```python
from build123d import *

# Parameters (mm, degrees)
F0_W        = 50.8
F0_H        = 26.0105735242
F1_DEPTH    = 6.35
F2_W        = 50.6046172231
F2_H        = 51.1175021529
F3_DEPTH    = 25.4
F4_T4_DEPTH = 51.1175021529
F4_T9_DEPTH = 64.038633205
F5_SIZE     = 5.08


# Not quite as in the source:
# - a fillet or chamfer that OpenCascade refuses, or shapes differently, is made with other operations: its cross-section is extruded or revolved along the edge and cut away or added


with BuildPart() as f1:
    # F0 (on Front) → F1 (new body)
    with BuildSketch(Plane.XZ):
        with Locations((0, -37.7947132379)):
            Rectangle(F0_W, F0_H)
        Polygon((-38.1, -24.7894264758), (-25.4, -24.7894264758), (-25.4, 0), align=None)
        Polygon((25.4, -50.8), (-25.4, -50.8), (-25.4, -24.7894264758), (-38.1, -24.7894264758), (-38.1, -51.4594204724), (38.1, -51.4594204724), (38.1, -24.7894264758), (25.4, -24.7894264758), align=None)
        Polygon((25.4, 0), (25.4, -24.7894264758), (38.1, -24.7894264758), align=None)
        Polygon((-25.4, 0), (-25.4, -24.7894264758), (25.4, -24.7894264758), (25.4, 0), (25.4, 50.8), (-25.4, 50.8), align=None)
    extrude(amount=F1_DEPTH)

    # F2 (on Front) → F3 (join)
    with BuildSketch(Plane.XZ):
        with Locations((-0.1709619537, -25.5587510765)):
            Rectangle(F2_W, F2_H)
    extrude(amount=F3_DEPTH)

    # F4: chamfer of 5.08 on 2 edges, made by hand


with BuildPart() as f4_tool2:
    # F4_s3 → F4_t4 (new body)
    with BuildSketch(Plane.XY):
        Polygon((30.2113466579, -6.35), (25.1313466579, -11.43), (25.1313466579, -6.35), align=None)
    extrude(amount=-F4_T4_DEPTH)

    split(bisect_by=Plane(origin=(20.1193399264, 0, 10.3074436722), x_dir=(0, 1, 0), z_dir=(-0.8899999984, 0, -0.4559605278)), keep=Keep.TOP)


with BuildPart() as f1_1:
    add(f1.part)

    # F4_t1: union F4_tool2
    add(f4_tool2.part)


with BuildPart() as f4_tool7:
    # F4_s8 → F4_t9 (new body)
    with BuildSketch(Plane.XY.offset(-51.1175021529)):
        Polygon((-25.4732705653, -11.43), (-30.5532705653, -6.35), (-25.4732705653, -6.35), align=None)
    extrude(amount=F4_T9_DEPTH)

    split(bisect_by=Plane(origin=(-20.1193399264, 0, 10.3074436722), x_dir=(0, 1, 0), z_dir=(0.8899999984, 0, -0.4559605278)), keep=Keep.TOP)


with BuildPart() as f1_2:
    add(f1_1.part)

    # F4_t6: union F4_tool7
    add(f4_tool7.part)

    # F5
    f5_edges = [f1_2.edges().sort_by_distance(p)[0] for p in [
        (25.131347, -11.43, -25.558751),
        (-25.473271, -11.43, -25.63026),
    ]]
    chamfer(f5_edges, length=F5_SIZE)


solid = f1_2.part
```
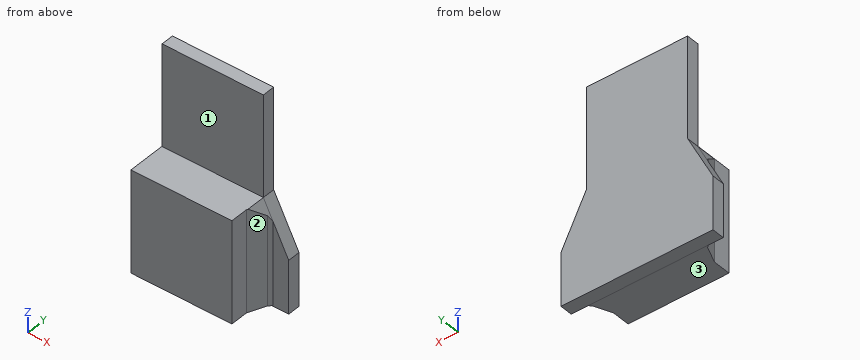
Read the model definition and answer for the solid it produces. Units are mm, in the model's axes. Face numbers are marked on the shaded views. A direction names the side the tool comes from. Round coordinates to 2 decimals unless told otherwise and drop trailing zeros. Write each loop counter-clockwise with the first axis right and the second up, starting at its lowest first coordinate (ties: lowest second). Pieces come first, ordered by that corner, then holes. Notation, with made-up numbers: (12.5, -20) - (37.5, -20) arc R24 ccw to (37.5, -5) - close; hole circle Ø7 at (-24.75, -28). An arc over 180 degrees is marked (long way). One line per item, written item: value.
Q1. Which of the six approach directions +Z, -Z, +X, -X, +Y, -Y give full straight-line access (tool end or side, diameter ignored) to the marked faces 1, 2 and 3?
The answers:
face 1: +Z, +X, -X, -Y
face 2: +Z, -Z, +X, -Y
face 3: -Z, +X, -X, -Y
Q2. Find section C-C (y = -21.5). Determine the outline of the cut face in (x, z).
The answers:
outline: (-25.47, -51.12) - (25.13, -51.12) - (25.13, 0) - (-25.47, 0) - close
Q3. Find section A-A (z = -32). Determine the outline of the cut face in (x, y), and give its area (3 significant figures).
The answers:
outline: (-38.1, -6.35) - (-30.55, -6.35) - (-29.07, -7.84) - (-25.47, -16.51) - (-25.47, -25.4) - (25.13, -25.4) - (25.13, -16.51) - (28.72, -7.84) - (30.21, -6.35) - (38.1, -6.35) - (38.1, 0) - (-38.1, 0) - close
area: 1,490 mm2
Q4. Find section B-B (x = 7.5). Determine the outline of the cut face in (y, z).
The answers:
outline: (-25.4, -51.12) - (-6.35, -51.12) - (-6.35, -51.46) - (0, -51.46) - (0, 50.8) - (-6.35, 50.8) - (-6.35, 0) - (-25.4, 0) - close
Q5. Straight lines are drawn through the part: line 1 (Y direction, x = 7.5, z = 6); line 2 (Z direction, x = 9, y = -9). For each, find the intervals that lie inside material, in ascending order. Write a range as from..to.
The answers:
line 1: y = -6.35..0
line 2: z = -51.12..0
Q6. Find section D-D (z = -18). Determine the outline of the cut face in (x, y), and give its area (3 significant figures).
The answers:
outline: (-34.62, -6.35) - (-30.55, -6.35) - (-29.07, -7.84) - (-25.47, -16.51) - (-25.47, -25.4) - (25.13, -25.4) - (25.13, -16.51) - (28.72, -7.84) - (30.21, -6.35) - (34.62, -6.35) - (34.62, 0) - (-34.62, 0) - close
area: 1,450 mm2
Q7. Each of these flat-tipped pins is pushed along its axis until it touches: P1, Ø6, axis at y = -13.5, z = -1, coming from the -X side; P2, Ø3, axis at x = 26.5, y = -8, coming from the -Z side; P3, Ø10, axis at y = -21, z = -36.5, coming from the +X side. Where does it stop, or does it pass through?
The answers:
P1: stops at x = -27.28
P2: stops at z = -51.12
P3: stops at x = 25.34
